Part model, mm, in its own coordinate system. Face numbers are marked on the shaded views. A direction names the side the tool comes from. Coordinates: 2 decimals unless noted, no trailing zeros. Loops run counter-clockwise (first coordinate to the right, second up) from the corner with the lowest first, then second, coordinate; pieces in that order, holes last. Notation, with made-up numbers: (84.5, 52.25) -> (140.5, 52.25) arc R22 cw to (140.5, 68.25) -> close; hole circle Ø10 at (-23, 51). An arc over 180 degrees is marked (long way). Use one line per item in the form item = value. Start each with the question number.
(1) 3-axis set-ups, long thin cutter, end or side, ignore diameter. For the marked faces 1, 2 and 3: which of +Z, -Z, +X, -X, +Y, -Y reach the whole face in a straight line?
(2) Band-saw the part on A-A on z = 8.5. Give the cut face in (x, y), then the cut area to 3 significant figures.
(3) Drill centre lines: L1, parallel to X at y = 0.5, z = 0; L2, parallel to Y at x = -8.85, z = 0.5; L3, parallel to Z at x = 3, y = 10. Where is each one in solid material? Low to high. Write a range as [from, to].
(4) Band-saw the part on C-C on z = 0. Give the cut face in (x, y).
(5) Band-saw the part on B-B on x = -35. Give the cut face in (y, z), then the cut area to 3 significant figures.
(6) Pin check, flat tips, straight feed: P1, Ø1.6, axis at x = -8.5, y = 54, coming from the +Z side; P2, Ø1.6, axis at x = -9.5, y = 55.5, coming from the -Z side; P3, Ø2, axis at y = 51.5, z = -16.5, coming from the -X side; P4, Ø16, axis at x = 35, z = 0, coming from the -Y side. Stop position of each tip, or through.
(7) Band-saw the part on D-D on y = 49. Give the cut face in (x, z).
(8) Mould opens along Z. For the marked faces 4, 5 and 6 say: +Z half, -Z half, draft (parallel to the pull), parting line (faces both ways), or undercut.
```python
from build123d import *

# Parameters (mm, degrees)
CROQUIS1_W              = 100
CROQUIS1_H              = 55
SALIENTE_EXTRUIR1_DEPTH = 2
CROQUIS2_R              = 5
CORTAR_EXTRUIR1_DEPTH   = 2
SALIENTE_EXTRUIR2_DEPTH = 65
CORTAR_EXTRUIR2_DEPTH   = 55
REDONDEO1_R             = 5
CROQUIS6_R              = 1.9
CORTAR_EXTRUIR3_DEPTH   = 2


with BuildPart() as part:
    # Croquis1 → Saliente-Extruir1 (new body)
    with BuildSketch(Plane(origin=(0, 0, 0), x_dir=(1, 0, 0), z_dir=(0, 1, 0))):
        Rectangle(CROQUIS1_W, CROQUIS1_H)
    extrude(amount=SALIENTE_EXTRUIR1_DEPTH)

    # Croquis2 → Cortar-Extruir1 (cut)
    with BuildSketch(Plane(origin=(0, 2, 0), x_dir=(1, 0, 0), z_dir=(0, 1, 0))):
        with Locations((35, 0)):
            Circle(CROQUIS2_R)
        with Locations((-35, 0)):
            Circle(CROQUIS2_R)
    extrude(amount=-CORTAR_EXTRUIR1_DEPTH, mode=Mode.SUBTRACT)

    # Croquis3 → Saliente-Extruir2 (add)
    with BuildSketch(Plane(origin=(0, 2, 0), x_dir=(1, 0, 0), z_dir=(0, 1, 0))):
        with BuildLine():
            Line((30, 27.5), (-7, 27.5))
            ThreePointArc((-7, 27.5), (-9.121320344, 26.621320344), (-10, 24.5))
            Line((-10, 24.5), (-10, -24.5))
            ThreePointArc((-10, -24.5), (-9.121320344, -26.621320344), (-7, -27.5))
            Line((-7, -27.5), (30, -27.5))
            Line((30, -27.5), (30, -25.5))
            Line((30, -25.5), (-7, -25.5))
            ThreePointArc((-7, -25.5), (-7.707106781, -25.207106781), (-8, -24.5))
            Line((-8, -24.5), (-8, 24.5))
            ThreePointArc((-8, 24.5), (-7.707106781, 25.207106781), (-7, 25.5))
            Line((-7, 25.5), (30, 25.5))
            Line((30, 25.5), (30, 27.5))
        make_face()
    extrude(amount=SALIENTE_EXTRUIR2_DEPTH)

    # Croquis4 → Cortar-Extruir2 (cut)
    with BuildSketch(Plane.XY.offset(27.5)):
        Polygon((-8, 67), (30, 2), (30, 67), align=None)
    extrude(amount=-CORTAR_EXTRUIR2_DEPTH, mode=Mode.SUBTRACT)

    # Redondeo1
    redondeo1_edges = [part.edges().sort_by_distance(p)[0] for p in [
        (50, 1, 27.5),
        (-50, 1, 27.5),
        (-50, 1, -27.5),
        (50, 1, -27.5),
    ]]
    fillet(redondeo1_edges, radius=REDONDEO1_R)

    # Croquis6 → Cortar-Extruir3 (cut)
    with BuildSketch(Plane(origin=(-8, 0, 0), x_dir=(0, 0, -1), z_dir=(1, 0, 0))):
        with Locations((-8.5, 41.9)):
            Circle(CROQUIS6_R)
        with Locations((-0.5, 33.9)):
            Circle(CROQUIS6_R)
        with Locations((7.5, 41.9)):
            Circle(CROQUIS6_R)
        with BuildLine():
            Line((-6, 41.9), (-6, 67))
            Line((-6, 67), (5, 67))
            Line((5, 67), (5, 41.9))
            ThreePointArc((5, 41.9), (-0.5, 36.4), (-6, 41.9))
        make_face()
    extrude(amount=-CORTAR_EXTRUIR3_DEPTH, mode=Mode.SUBTRACT)


solid = part.part
```
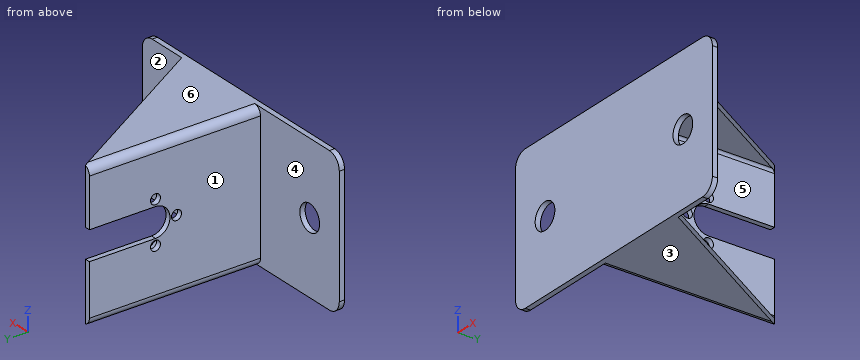
A:
q1.face_1 = +Z, -Z, -X, +Y
q1.face_2 = +X, +Y
q1.face_3 = -Z, +X, -X, +Y, -Y
q2.outline = (-50, 0) -> (50, 0) -> (50, 2) -> (-8, 2) -> (-8, 40) -> (-10, 40) -> (-10, 2) -> (-50, 2) -> close; (-10, 43.8) -> (-8, 43.8) -> (-8, 67) -> (-10, 67) -> close
q2.area = 322 mm²
q3.L1 = [-50, -40], [-30, 30], [40, 50]
q3.L2 = [0, 32], [35.8, 36.4]
q3.L3 = [-27.5, -25.5], [25.5, 27.5]
q4.outline = (-50, 0) -> (-40, 0) -> (-40, 2) -> (-50, 2) -> close; (-30, 0) -> (30, 0) -> (30, 2) -> (-8, 2) -> (-8, 32.07) -> (-10, 32.07) -> (-10, 2) -> (-30, 2) -> close; (-10, 35.73) -> (-8, 35.73) -> (-8, 36.42) -> (-10, 36.42) -> close; (40, 0) -> (50, 0) -> (50, 2) -> (40, 2) -> close
q5.outline = (0, -27.5) -> (2, -27.5) -> (2, -5) -> (0, -5) -> close; (0, 5) -> (2, 5) -> (2, 27.5) -> (0, 27.5) -> close
q5.area = 90.0 mm²
q6.P1 = 27.42
q6.P2 = -26.97
q6.P3 = -10
q6.P4 = 0
q7.outline = (-10, -24.5) arc R3 ccw to (-7, -27.5) -> (2.52, -27.5) -> (2.52, -25.5) -> (-7, -25.5) arc R1 cw to (-8, -24.5) -> (-8, -5) -> (-10, -5) -> close; (-10, 6) -> (-8, 6) -> (-8, 24.5) arc R1 cw to (-7, 25.5) -> (2.52, 25.5) -> (2.52, 27.5) -> (-7, 27.5) arc R3 ccw to (-10, 24.5) -> close
q8.face_4 = draft
q8.face_5 = undercut
q8.face_6 = +Z half
